from build123d import *

# Parameters (mm, degrees)
F0_W      = 60
F0_H      = 80
F1_DEPTH  = 20
F2_W      = 80
F2_H      = 90
F3_DEPTH  = 25
F4_R      = 3
F5_DEPTH  = 25.001
F6_W      = 20
F6_H      = 60
F7_DEPTH  = 55
F8_W      = 40
F8_H      = 40
F8_W_2    = 5
F8_H_2    = 12
F8_W_3    = 12
F8_H_3    = 5
F9_DEPTH  = 68.001
F10_R     = 3
F11_DEPTH = 75.001
F12_R     = 3
F13_DEPTH = 3


with BuildPart() as f1:
    # F0 (on Right) → F1 (new body)
    with BuildSketch(Plane.YZ):
        Rectangle(F0_W, F0_H)
    extrude(amount=F1_DEPTH)

    # F2 (on face) → F3 (join)
    with BuildSketch(Plane(origin=(0, 0, -40), x_dir=(1, 0, 0), z_dir=(0, 0, -1))):
        with Locations((-20, 0)):
            Rectangle(F2_W, F2_H)
    extrude(amount=-F3_DEPTH)

    # F4 (on face) → F5 (cut, through all)
    with BuildSketch(Plane.XY.offset(-15)):
        with Locations((-48, 37)):
            Circle(F4_R)
        with Locations((-48, -37)):
            Circle(F4_R)
        with Locations((8, -37)):
            Circle(F4_R)
        with Locations((8, 37)):
            Circle(F4_R)
    extrude(amount=-F5_DEPTH, mode=Mode.SUBTRACT)

    # F6 (on face) → F7 (join, through all)
    with BuildSketch(Plane.XY.offset(-15)):
        with Locations((-38, 0)):
            Rectangle(F6_W, F6_H)
    extrude(amount=F7_DEPTH)

    # F8 (on face) → F9 (cut, through all)
    with BuildSketch(Plane(origin=(-48, 0, 0), x_dir=(0, -1, 0), z_dir=(-1, 0, 0))):
        with Locations((0, 10)):
            Rectangle(F8_W, F8_H)
        with Locations((-24.5, 12.5)):
            Rectangle(F8_W_2, F8_H_2)
        with Locations((0, 34.5)):
            Rectangle(F8_W_3, F8_H_3)
        with Locations((24.5, 12.5)):
            Rectangle(F8_W_2, F8_H_2)
    extrude(amount=-F9_DEPTH, mode=Mode.SUBTRACT)

    # F10 (on face) → F11 (cut, through all)
    with BuildSketch(Plane.XZ.offset(30)):
        with Locations((-38, 12.5)):
            Circle(F10_R)
        with Locations((10, 12.5)):
            Circle(F10_R)
    extrude(amount=-F11_DEPTH, mode=Mode.SUBTRACT)

    # F12 (on face) → F13 (cut, through all)
    with BuildSketch(Plane.XY.offset(40)):
        with Locations((-38, 0)):
            Circle(F12_R)
        with Locations((10, 0)):
            Circle(F12_R)
    extrude(amount=-F13_DEPTH, mode=Mode.SUBTRACT)


solid = f1.part
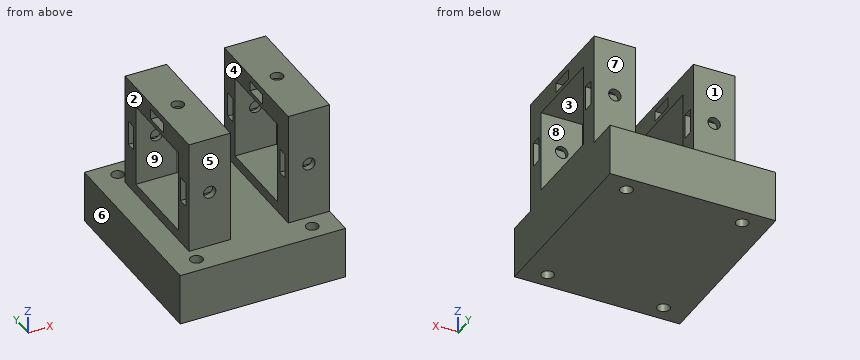
Could you check a few things on this model? Use its own coordinates, in mm. Face numbers are marked on the shaded views. A direction names the side the tool comes from. Round coordinates to 2 decimals unless told otherwise and drop trailing zeros. Order: outer loops, then holes, each group sorted by start corner. A loop starts at its lowest first (then second) coordinate and runs counter-clockwise, first axis right, second up.
(1) If we mould it in two halves opening along Y, with no side actions, what happens to the marked faces 6, 7, 8 and 9? For each: released by +Y, released by -Y, zero draft, split by the parting line, or undercut.
Response values:
face 6: zero draft
face 7: released by +Y
face 8: undercut
face 9: undercut
(2) Imagine slicing it at B-B (y = 0). Count the separate pieces of the cut face and the enclosed holes in it, plus the area to 3 significant figures.
Response values:
separate pieces: 7
enclosed holes: 0
area: 2,360 mm2
(3) Imagine slicing it at A-A (z = -12). Write out the boundary of the cut face in (x, y), plus the area to 3 significant figures.
Response values:
outline: (-48, -30) - (-28, -30) - (-28, 30) - (-48, 30) - close; (0, -30) - (20, -30) - (20, 30) - (0, 30) - close
area: 2,400 mm2
(4) I'm going to push flat-ended pins straight in: pin 1 (10 mm diameter, centred on x = -37, z = 6.5, fed in from -Y); pin 2 (1.5 mm diameter, centred on x = -26, z = 3.5, fed in from +Y); pin 3 (9.5 mm diameter, centred on x = -33, z = 13.5, fed in from +Y); pin 4 (16.5 mm diameter, centred on y = -12.5, z = 8, fed in from -X). Where does each tip first touch, or does it pass through?
Response values:
pin 1: stops at y = -30
pin 2: passes through
pin 3: stops at y = 30
pin 4: stops at x = -48
(5) Which directions (+Z, -Z, +X, -X, +Y, -Y) give clear straight access to the entire face, cutting with the end or side of a thin tool? Please do the marked faces 1, 2, 3, 4 and 5.
Response values:
face 1: +Z, +X, -X, +Y
face 2: +Z, -X, +Y, -Y
face 3: +X, -X
face 4: +Z, +Y, -Y
face 5: +Z, +X, -X, -Y
(6) Please list where these lines run through material, in increasing order: line 1 along Y through (x, z) = (8, -31); line 2 along Y through (x, z) = (-47, 8); line 3 along Z through (x, y) = (-38, -28).
Response values:
line 1: y = -45 to -40, -34 to 34, 40 to 45
line 2: y = -30 to -27, -22 to -20, 20 to 22, 27 to 30
line 3: z = -40 to 9.5, 15.5 to 40
(7) Imagine slicing it at D-D (z = -34). Write out the boundary of the cut face in (x, y), plus the area to 3 significant figures.
Response values:
outline: (-60, -45) - (20, -45) - (20, 45) - (-60, 45) - close; hole circle Ø6 at (-48, -37); hole circle Ø6 at (-48, 37); hole circle Ø6 at (8, -37); hole circle Ø6 at (8, 37)
area: 7,090 mm2
(8) Imagine slicing it at C-C (y = 37). Write out the boundary of the cut face in (x, z), plus the area to 3 significant figures.
Response values:
outline: (-60, -40) - (-51, -40) - (-51, -15) - (-60, -15) - close; (-45, -40) - (5, -40) - (5, -15) - (-45, -15) - close; (11, -40) - (20, -40) - (20, -15) - (11, -15) - close
area: 1,700 mm2
